from build123d import *

# Parameters (mm, degrees)
SKETCH068_W     = 12
SKETCH068_H     = 8
PAD060_DEPTH    = 24.25
SKETCH069_R     = 3
SKETCH069_R_2   = 1
PAD061_DEPTH    = 5.9
SKETCH071_R     = 1.55
POCKET_DEPTH    = 8.001
POCKET001_DEPTH = 3
SKETCH072_W     = 11
SKETCH072_H     = 24.25
PAD062_DEPTH    = 3


with BuildPart() as front_axle_right:
    # Sketch068 → Pad060 (new body)
    with BuildSketch(Plane.YZ):
        with Locations((38, -7.15)):
            Rectangle(SKETCH068_W, SKETCH068_H)
    extrude(amount=PAD060_DEPTH)

    # Sketch069 (on Face6 of Pad060) → Pad061 (join)
    with BuildSketch(Plane.YZ.offset(24.25)):
        with Locations((38, -7.8)):
            Circle(SKETCH069_R)
        with Locations((38, -7.8)):
            Circle(SKETCH069_R_2, mode=Mode.SUBTRACT)
    extrude(amount=PAD061_DEPTH)

    # Sketch071 (on Face1 of Pad061) → Pocket (cut, through all)
    with BuildSketch(Plane(origin=(0, 0, -3.15), x_dir=(0, -1, 0), z_dir=(0, 0, 1))):
        with Locations((-38, 10)):
            Circle(SKETCH071_R)
    extrude(amount=-POCKET_DEPTH, mode=Mode.SUBTRACT)

    # Sketch070 (on Face1 of Pocket) → Pocket001 (cut)
    with BuildSketch(Plane(origin=(0, 0, -3.15), x_dir=(0, -1, 0), z_dir=(0, 0, 1))):
        Polygon((-34.709103, 10), (-36.354552, 12.85), (-39.645448, 12.85), (-41.290897, 10), (-39.645448, 7.15), (-36.354552, 7.15), align=None)
    extrude(amount=-POCKET001_DEPTH, mode=Mode.SUBTRACT)

    # Sketch072 (on Face5 of Pocket001) → Pad062 (join)
    with BuildSketch(Plane.ZX.offset(44)):
        with Locations((-8.65, 12.125)):
            Rectangle(SKETCH072_W, SKETCH072_H)
    extrude(amount=PAD062_DEPTH)


with BuildPart() as front_axle_right_mirrored:
    # Mirror: instance of front_axle_right
    add(front_axle_right.part.mirror(Plane(origin=(3e-06, 39.5, -8.649999), x_dir=(0, -1, 0), z_dir=(1, 0, 0))))


solid = front_axle_right_mirrored.part
Could you check a few things on this model? Use its own coordinates, in mm. A direction names the side the tool comes from. Give positions to 0.01 mm unless a question says otherwise; leave off trailing zeros. Write each loop counter-clockwise with the first axis right and the second up, starting at its lowest first coordinate (ties: lowest second). Pieces come first, ordered by that corner, then holes. Notation, with made-up numbers: (22, 0.25) -> (32, 0.25) arc R25 cw to (32, 19.25) -> close; hole circle Ø3 at (49.5, 36). An arc over 180 degrees is marked (long way). Write each question's results on one line, items separated by ' | '. Start each with the question number.
Q1. Suppose I cut it at D-D, the plane x = -25.5. List the corners of the cut face in (y, z) for me.
Q2. Suppose I cut it at A-A, the plane z = -7.8. List the corners of the cut face in (x, y) for me.
Q3. I need wall thicknesses on probe 1 along X at (y, z) = (38, -7.75); probe 2 along Z at (x, y) = (-2, 42.75); probe 3 along X at (y, z) = (38, -9.55). Which ranges of each line are inside material? Lowest first, please.
Q4. Suppose I cut it at C-C, the plane x = -22. List the corners of the cut face in (y, z) for me.
Q5. We'd pull the mould along Y, two halves only. Please class faces 4 (the face through (-10.466, 36.522, -8.615)), 5 (the face through (0, 39, -8)), 6 (the face through (-12, 47, -9)): +Y half, -Y half, draft (parallel to the pull), parting line (faces both ways), or undercut.
Q6. Which directions (+Z, -Z, +X, -X, +Y, -Y) give clear straight access to the entire face, cutting with the end or side of a thin tool? Please do faces 1 (the face through (-11.3, 36.6, -6.15)), 2 (the face through (-12, 38, -11.15)), 3 (the face through (-24.25, 38, -8)).
Q7. Suppose I cut it at B-B, the plane y = 38. List the corners of the cut face in (x, z) for me, and give its area (3 significant figures).
Q8. I'm going to push flat-ended pins straight in: pin 1 Ø3 at (x, y) = (-9.5, 38.5) entering from +Z; pin 2 Ø6 at (y, z) = (45, -5.5) entering from -X; pin 3 Ø3.5 at (x, y) = (-17, 37.5) entering from -Z. Where does each tip first touch, or does it pass through?
Outcome:
1) outline: circle Ø6 at (38, -7.8); hole circle Ø2 at (38, -7.8)
2) outline: (-30.15, 35) -> (-24.25, 35) -> (-24.25, 32) -> (0, 32) -> (0, 47) -> (-24.25, 47) -> (-24.25, 41) -> (-30.15, 41) -> (-30.15, 39) -> (-24.25, 39) -> (-24.25, 37) -> (-30.15, 37) -> close; hole circle Ø3.1 at (-10, 38)
3) probe 1: -24.25 to -11.55, -8.45 to 0 | probe 2: -11.15 to -3.15 | probe 3: -30.15 to -11.55, -8.45 to 0
4) outline: (32, -11.15) -> (44, -11.15) -> (44, -14.15) -> (47, -14.15) -> (47, -3.15) -> (32, -3.15) -> close
5) face 4: undercut | face 5: draft | face 6: +Y half
6) face 1: +Z | face 2: -Z, +X, -X, -Y | face 3: -X
7) outline: (-30.15, -10.8) -> (-24.25, -10.8) -> (-24.25, -11.15) -> (-11.55, -11.15) -> (-11.55, -6.15) -> (-12.85, -6.15) -> (-12.85, -3.15) -> (-24.25, -3.15) -> (-24.25, -4.8) -> (-30.15, -4.8) -> (-30.15, -6.8) -> (-24.25, -6.8) -> (-24.25, -8.8) -> (-30.15, -8.8) -> close; (-8.45, -11.15) -> (0, -11.15) -> (0, -3.15) -> (-7.15, -3.15) -> (-7.15, -6.15) -> (-8.45, -6.15) -> close | area: 185 mm2
8) pin 1: z = -6.15 | pin 2: x = -24.25 | pin 3: z = -11.15
